Can you work these out from the drawing? Everything is in mm from the part's minimum corner. A direction names the side the tool comes from. Give positions to 0.01 mm unless a question says otherwise; leave off trailing zeros. Order: outer loops, then holes, each group sorted by start corner. A loop starts at its lowest first (then second) coordinate and runs counter-clockwise, first axis right, second up. Notation, with made-up numbers: (61, -16.75) - (103, -16.75) arc R7 ccw to (103, -7.75) - close; hole circle Ø5 at (-14.75, 46). An arc over 180 degrees is marked (long way). One line per question, with ' | ' between items.
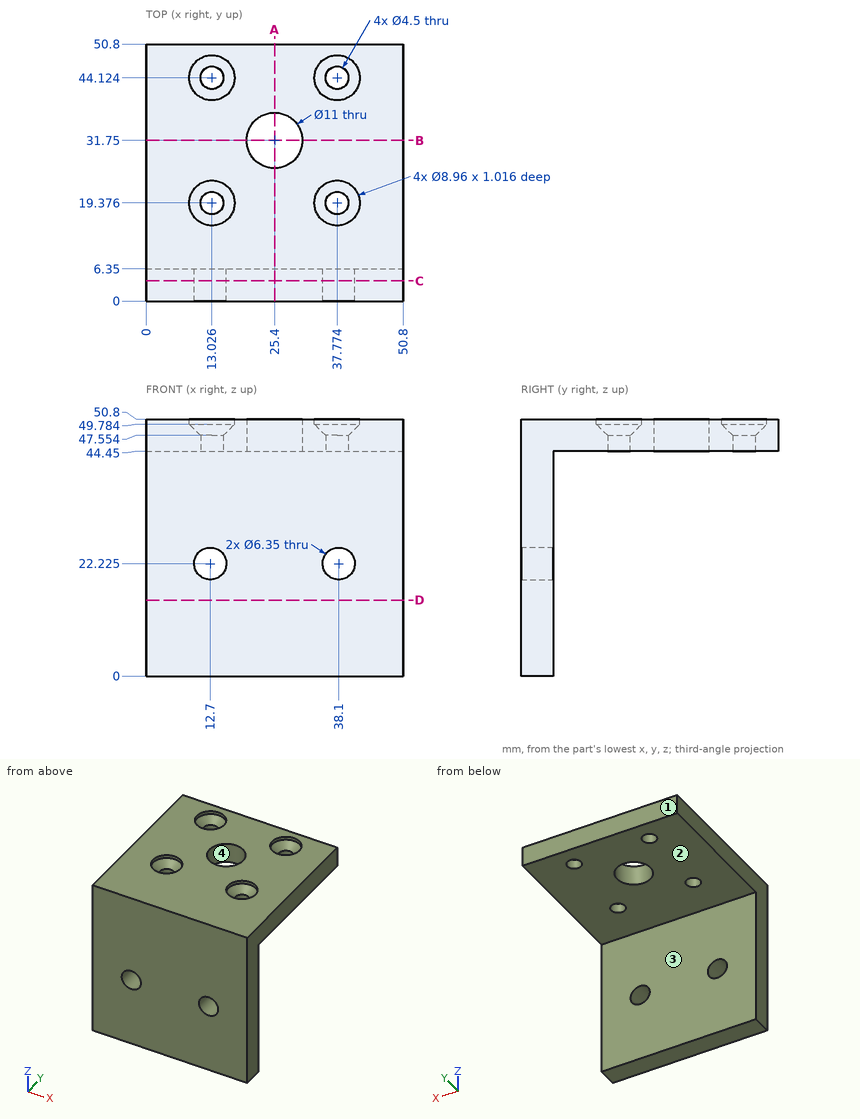
1) Thinking about a two-plate mould opening in X: for the marked faces 3 and 4, which applies, +X half, -X half, draft (parallel to the pull), parting line (faces both ways), or undercut?
Model answer:
face 3: draft | face 4: undercut
2) I want a section at D-D (z = 15). List the corners of the cut face in (x, y) for me.
Model answer:
outline: (0, 0) - (50.8, 0) - (50.8, 6.35) - (0, 6.35) - close
3) I want a section at C-C (y = 4). State how many separate pieces and enclosed holes the cut face has, plus the area to 3 significant figures.
Model answer:
separate pieces: 1 | enclosed holes: 2 | area: 2,520 mm2
4) Please list where these lines run through material, in increasing order: L1, parallel to Y at x = 26, z = 40.5; L2, parallel to Z at x = 38, y = 34; L3, parallel to Y at x = 15, z = 47.5 (1 decimal).
Model answer:
L1: y = 0 to 6.35 | L2: z = 44.45 to 50.8 | L3: y = 0 to 18.3, 20.5 to 43, 45.2 to 50.8
5) I'm going to push flat-ended pins straight in: P1, Ø3, axis at x = 32, y = 8, coming from the -Z side; P2, Ø3, axis at x = 34, z = 40, coming from the +Y side; P3, Ø7, axis at x = 37.77, y = 19.38, coming from the +Z side. Where does each tip first touch, or does it pass through?
Model answer:
P1: stops at z = 44.45 | P2: stops at y = 6.35 | P3: stops at z = 48.81
6) I want a section at B-B (y = 31.75). List the corners of the cut face in (x, z) for me, plus the area to 3 significant figures.
Model answer:
outline: (0, 44.45) - (19.9, 44.45) - (19.9, 50.8) - (0, 50.8) - close; (30.9, 44.45) - (50.8, 44.45) - (50.8, 50.8) - (30.9, 50.8) - close | area: 253 mm2
7) On a 3-axis mill with a long thin cutter (end or side, diameter ignored), from which of +Z, -Z, +X, -X, +Y, -Y can I reach the whole of each face in a straight line? I mean the marked faces 1 and 2. Say none if no direction works.
Model answer:
face 1: +Z, -Z, +X, -X, +Y | face 2: -Z, +X, -X, +Y
8) I want a section at A-A (x = 25.4). List the corners of the cut face in (y, z) for me, plus the area to 3 significant figures.
Model answer:
outline: (0, 0) - (6.35, 0) - (6.35, 44.45) - (26.25, 44.45) - (26.25, 50.8) - (0, 50.8) - close; (37.25, 44.45) - (50.8, 44.45) - (50.8, 50.8) - (37.25, 50.8) - close | area: 535 mm2
